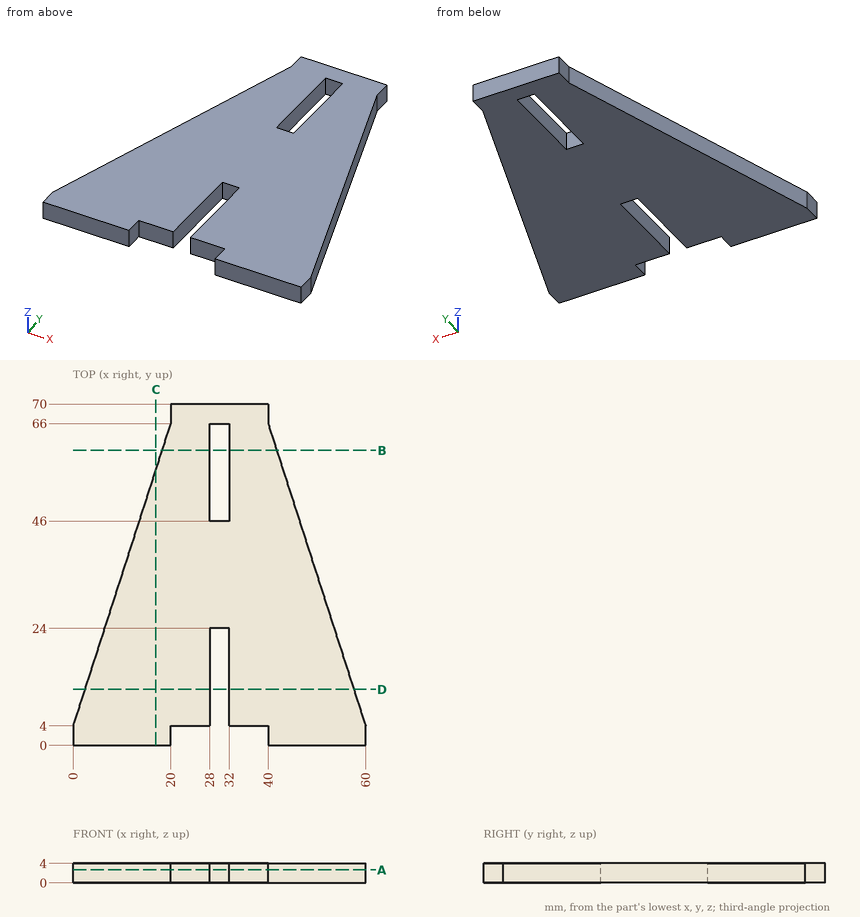
Job drawing, mm, ordinate dimensions from the low corner. One solid piece. Round coordinates to 2 decimals unless told otherwise and drop trailing zeros. Order: outer loops, then holes, each group sorted by start corner. A loop starts at its lowest first (then second) coordinate and runs counter-clockwise, first axis right, second up. Notation, with made-up numbers: (17.5, 76) - (60.5, 76) arc R20 cw to (60.5, 84) - close; hole circle Ø9 at (25.25, 75.25). An arc over 180 degrees is marked (long way). Use CSV: the item, a comma, the result in double quotes. Start each with the question number.
1) Saw through at C-C (x = 17). List the corners of the cut face in (y, z), and give its area (3 significant figures).
2) Pin check, flat tips, straight feed: pin 1 Ø2 at (y, z) = (52.5, 1) entering from +X; pin 2 Ø1.2 at (y, z) = (9.5, 3) entering from +X; pin 3 Ø2 at (x, z) = (37, 2.5) entering from -Y; pin 4 Ø8 at (x, y) = (38.5, 53) entering from -Z. Stop position of each tip, or through.
3) Saw through at B-B (y = 60.5). List the corners of the cut face in (x, z).
4) Saw through at A-A (z = 2.65). List the corners of the cut face in (x, y).
5) Saw through at D-D (y = 11.5). List the corners of the cut face in (x, z), and give its area (3 significant figures).
6) Wall check: L1, parallel to Y at x = 36, z = 0.35; L2, parallel to X at y = 7.5, z = 2.8; L3, parallel to Y at x = 29.5, z = 3.8. Give the ranges that are in metal, low to high. Write a range as [from, to].
Values follow:
1,outline,"(0, 0) - (56.7, 0) - (56.7, 4) - (0, 4) - close"
1,area,"227 mm2"
2,pin 1,"stops at x = 44.68"
2,pin 2,"stops at x = 58.42"
2,pin 3,"stops at y = 4"
2,pin 4,"stops at z = 0"
3,outline,"(18.23, 0) - (28, 0) - (28, 4) - (18.23, 4) - close; (32, 0) - (41.77, 0) - (41.77, 4) - (32, 4) - close"
4,outline,"(0, 0) - (20, 0) - (20, 4) - (28, 4) - (28, 24) - (32, 24) - (32, 4) - (40, 4) - (40, 0) - (60, 0) - (60, 4) - (40, 66) - (40, 70) - (20, 70) - (20, 66) - (0, 4) - close; hole (28, 46) - (32, 46) - (32, 66) - (28, 66) - close"
5,outline,"(2.42, 0) - (28, 0) - (28, 4) - (2.42, 4) - close; (32, 0) - (57.58, 0) - (57.58, 4) - (32, 4) - close"
5,area,"205 mm2"
6,L1,"y = [4, 70]"
6,L2,"x = [1.13, 28], [32, 58.87]"
6,L3,"y = [24, 46], [66, 70]"
